```python
from build123d import *

# Parameters (mm, degrees)
BOSS_EXTRUDE1_DEPTH   = 11.8
BOSS_EXTRUDE2_DEPTH   = 4
SKETCH4_R             = 2.3
BOSS_EXTRUDE3_DEPTH   = 3.2
SKETCH5_R             = 0.85
CUT_EXTRUDE1_DEPTH    = 1
CUT_EXTRUDE2_DEPTH    = 10
MOVER_START           = 28.4
MOVER_FACE2_OUTLINE_R = 2.3
MOVER_FACE2_DEPTH     = 1.9


# Read off the part's stored shape, not the designer's step: Mover face2
with BuildPart() as part:
    # Sketch2 → Boss-Extrude1 (new body)
    with BuildSketch(Plane(origin=(0, 0, 0), x_dir=(0, 0, -1), z_dir=(1, 0, 0))):
        Polygon((7.432291728, 0), (29.932291728, 0), (29.932291728, 15.9), (34.632291728, 15.9), (34.632291728, 18.4), (29.932291728, 18.4), (29.932291728, 23.1), (6.982957442, 23.1), (6.982957442, 18.4), (2.282957442, 18.4), (2.282957442, 15.9), (7.432291728, 15.9), align=None)
    extrude(amount=BOSS_EXTRUDE1_DEPTH)

    # Sketch3 → Boss-Extrude2 (add)
    with BuildSketch(Plane(origin=(0, 23.1, 0), x_dir=(-1, 0, 0), z_dir=(0, 1, 0))):
        with BuildLine():
            Line((-3.4, -16.098037438), (-3.4, -18.753881751))
            ThreePointArc((-3.4, -18.753881751), (-5.9, -29.998037438), (-8.4, -18.753881751))
            Line((-8.4, -18.753881751), (-8.4, -16.098037438))
            ThreePointArc((-8.4, -16.098037438), (-5.9, -13.598037438), (-3.4, -16.098037438))
        make_face()
    extrude(amount=BOSS_EXTRUDE2_DEPTH)

    # Sketch4 → Boss-Extrude3 (add)
    with BuildSketch(Plane(origin=(0, 27.1, 0), x_dir=(-1, 0, 0), z_dir=(0, 1, 0))):
        with Locations(Location((-5.9, -24.098037438, 0), (0, 0, 90))):
            Circle(SKETCH4_R)
    extrude(amount=BOSS_EXTRUDE3_DEPTH)

    # Sketch5 → Cut-Extrude1 (cut)
    with BuildSketch(Plane(origin=(0, 30.3, 0), x_dir=(1, 0, 0), z_dir=(0, 1, 0))):
        with Locations(Location((5.9, 24.098037438, 0), (0, 0, 270))):
            Circle(SKETCH5_R)
    extrude(amount=-CUT_EXTRUDE1_DEPTH, mode=Mode.SUBTRACT)

    # Sketch6 → Cut-Extrude2 (cut)
    with BuildSketch(Plane(origin=(0, 18.4, 0), x_dir=(1, 0, 0), z_dir=(0, 1, 0))):
        with BuildLine():
            Line((6.55, 2.282957442), (5.25, 2.282957442))
            Line((5.25, 2.282957442), (5.25, 3.823023234))
            ThreePointArc((5.25, 3.823023234), (5.9, 5.582957442), (6.55, 3.823023234))
            Line((6.55, 3.823023234), (6.55, 2.282957442))
        make_face()
        with BuildLine():
            Line((6.55, 34.632291728), (5.25, 34.632291728))
            Line((5.25, 34.632291728), (5.25, 33.092225935))
            ThreePointArc((5.25, 33.092225935), (5.9, 31.332291728), (6.55, 33.092225935))
            Line((6.55, 33.092225935), (6.55, 34.632291728))
        make_face()
    extrude(amount=-CUT_EXTRUDE2_DEPTH, mode=Mode.SUBTRACT)

    # Mover face2 outline → Mover face2 (cut)
    with BuildSketch(Plane(origin=(0, 0, 0), x_dir=(1, 0, 0), z_dir=(0, 1, 0)).offset(MOVER_START)):
        with Locations((5.9, 24.098037438)):
            Circle(MOVER_FACE2_OUTLINE_R)
    extrude(amount=MOVER_FACE2_DEPTH, mode=Mode.SUBTRACT)


solid = part.part
```
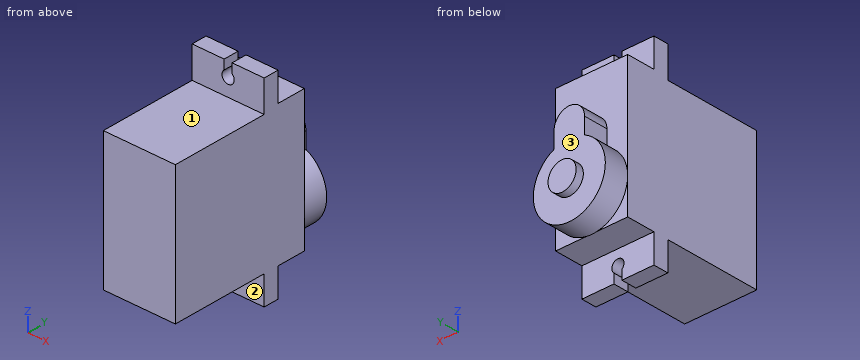
The listing builds one solid part. Answer for the finished solid, in the listing's coordinates (mm). Face numbers are marked on the shaded views. A direction names the side the tool comes from. Round coordinates to 2 decimals unless told otherwise and drop trailing zeros. Loops run counter-clockwise (first coordinate to the right, second up) from the corner with the lowest first, then second, coordinate; pieces in that order, holes last. Notation, with made-up numbers: (-22, -17) - (2, -17) arc R36 cw to (2, 22) - close; hole circle Ø5 at (0.5, -25). An arc over 180 degrees is marked (long way). Return JSON: item names as keys, results as strings. Group by question number.
1. The part is cut by section A-A on z = -18. Determine the outline of the cut face in (x, y), then the cut area to 3 significant figures.
2. Which of the six approach directions +Z, -Z, +X, -X, +Y, -Y give full straight-line access (tool end or side, diameter ignored) to the marked faces 1, 2 and 3?
3. The part is cut by section B-B on x = 5.9. Determine the outline of the cut face in (y, z), then the cut area to 3 significant figures.
4. Consider probe 1 along Y at (x, z) = (4.75, -14.5); probe 2 along Z at (x, y) = (3, 8.5); probe 3 along Y at (x, z) = (10.25, -15). Determine where each line is inside the solid, lowest interval first.
5. The part is cut by section C-C on y = 17.5. Determine the outline of the cut face in (x, z), then the cut area to 3 significant figures.
6. The part is cut by section D-D on z = -26. Determine the outline of the cut face in (x, y).
7. Each of these flat-tipped pins is pushed along its axis until it touches: P1, Ø3, axis at x = 5.9, z = -32.33, coming from the +Y side; P2, Ø3, axis at x = 10, y = 4, coming from the -Z side; P3, Ø5, axis at x = 5, z = -33, coming from the -Y side. Where does it stop, or does it pass through?
Resolved:
{
 "1": {"outline": "(0, 0) - (11.8, 0) - (11.8, 23.1) - (8.4, 23.1) - (8.4, 27.1) - (3.4, 27.1) - (3.4, 23.1) - (0, 23.1) - close", "area": "293 mm²"},
 "2": {"face 1": "+Z, +X, -X, -Y", "face 2": "-Z, +X, -X, -Y", "face 3": "+Y"},
 "3": {"outline": "(0, -29.93) - (15.9, -29.93) - (15.9, -31.33) - (18.4, -31.33) - (18.4, -29.93) - (23.1, -29.93) - (23.1, -30) - (27.1, -30) - (27.1, -26.4) - (28.4, -26.4) - (28.4, -21.8) - (27.1, -21.8) - (27.1, -13.6) - (23.1, -13.6) - (23.1, -6.98) - (18.4, -6.98) - (18.4, -5.58) - (15.9, -5.58) - (15.9, -7.43) - (0, -7.43) - close", "area": "602 mm²"},
 "4": {"probe 1": "y = 0 to 27.1", "probe 2": "z = -29.93 to -7.43", "probe 3": "y = 0 to 23.1"},
 "5": {"outline": "(0, -34.63) - (5.25, -34.63) - (5.25, -33.09) arc R1 cw (long way) to (6.55, -33.09) - (6.55, -34.63) - (11.8, -34.63) - (11.8, -2.28) - (6.55, -2.28) - (6.55, -3.82) arc R1 cw (long way) to (5.25, -3.82) - (5.25, -2.28) - (0, -2.28) - close", "area": "372 mm²"},
 "6": {"outline": "(0, 0) - (11.8, 0) - (11.8, 23.1) - (11.49, 23.1) - (11.49, 27.1) - (7.19, 27.1) - (7.19, 28.4) - (4.61, 28.4) - (4.61, 27.1) - (0.31, 27.1) - (0.31, 23.1) - (0, 23.1) - close"},
 "7": {"P1": "stops at y = 18.4", "P2": "stops at z = -29.93", "P3": "stops at y = 15.9"}
}
